from build123d import *

# Parameters (mm, degrees)
F0_W     = 152.4
F0_H     = 17.4625
F1_DEPTH = 8.73125
F3_DEPTH = 17.4625
F4_DEPTH = 17.4625


# Not quite as in the source:
# - a length typed as a fraction of an inch, garbled in the dataset ("3 / 203.2 mm" for 3/8 in), is restored


with BuildPart() as f1:
    # F0 (on Front) → F1 (new body, symmetric)
    with BuildSketch(Plane.XZ):
        Rectangle(F0_W, F0_H)
    extrude(amount=F1_DEPTH, both=True)

    # F2 (on face) → F3 (cut)
    with BuildSketch(Plane.XZ.offset(8.73125)):
        Polygon((-58.7375, -8.73125), (-76.2, 8.73125), (-76.2, -8.73125), align=None)
    extrude(amount=-F3_DEPTH, mode=Mode.SUBTRACT)

    # F2 (on face) → F4 (cut)
    with BuildSketch(Plane.XZ.offset(8.73125)):
        Polygon((76.2, -8.73125), (76.2, 8.73125), (58.7375, -8.73125), align=None)
    extrude(amount=-F4_DEPTH, mode=Mode.SUBTRACT)


solid = f1.part
Verification items for the finished model (mm, model axes). Coordinates: 2 decimals unless noted, no trailing zeros. Loops run counter-clockwise (first coordinate to the right, second up) from the corner with the lowest first, then second, coordinate; pieces in that order, holes last. Notation, with made-up numbers: (56, 73) -> (88, 73) arc R19 cw to (88, 103) -> close; hole circle Ø2 at (55, -37). An arc over 180 degrees is marked (long way). Write each question's results on one line, items separated by ' | '.
Item 1: Section check B-B, the plane z = 1.25. Enter the section's corners in (x, y), plus the area to 3 significant figures.
Found:
outline: (-68.72, -8.73) -> (68.72, -8.73) -> (68.72, 8.73) -> (-68.72, 8.73) -> close | area: 2,400 mm2
Item 2: Material ranges on L1, parallel to X at y = 3, z = -5.25; L2, parallel to X at y = 3.25, z = 1.75; L3, parallel to Z at x = 59.5, y = 7, recorded low to high.
Found:
L1: x = -62.22 to 62.22 | L2: x = -69.22 to 69.22 | L3: z = -7.97 to 8.73
Item 3: Gauge pin test, flat ends, axial feed: pin 1 (4 mm diameter, centred on y = 6, z = 3, fed in from -X); pin 2 (2 mm diameter, centred on y = -1.5, z = 1, fed in from +X); pin 3 (10 mm diameter, centred on y = 6, z = -3, fed in from -X). Record the tip position at first contact, or that the pin passes through.
Found:
pin 1: stops at x = -72.47 | pin 2: stops at x = 69.47 | pin 3: stops at x = -69.47
Item 4: Section check A-A, the plane y = -2.5. Enter the section's corners in (x, z).
Found:
outline: (-76.2, 8.73) -> (-58.74, -8.73) -> (58.74, -8.73) -> (76.2, 8.73) -> close
